Autodesk Inventor part; units mm, degrees
ref_plane "YZ Plane" through (0, 0, 0) normal (1, 0, 0) x (0, 1, 0)
ref_plane "XZ Plane" through (0, 0, 0) normal (0, 1, 0) x (-1, 0, 0)
ref_plane "XY Plane" through (0, 0, 0) normal (0, 0, 1) x (1, 0, 0)
sketch "Sketch1" plane through (0, 0, 0) normal (0, 1, 0) x (-1, 0, 0)
  line L0 (0, 0) -> (100, 0)
  line L1 (100, 0) -> (100, -180)
  line L2 (100, -180) -> (0, -180)
  line L3 (0, -180) -> (0, 0)
  dimension "d0" = 100
  dimension "d1" = 180
extrude "Extrusion1" add sketch "Sketch1" along normal blind 4
sketch "Sketch2" plane through (0, 4, 0) normal (0, 1, 0) x (1, 0, 0)
  line L0 (-100, 180) -> (-100, 0)
  line L1 (0, 180) -> (-100, 180)
  line L2 (-100, 0) -> (-96, 0)
  line L3 (-96, 0) -> (-96, 180)
  line L4 (-96, 180) -> (-100, 180)
  line L5 (-100, 180) -> (-100, 0)
  line L6 (0, 180) -> (-4, 180)
  line L7 (-4, 180) -> (-4, 0)
  line L8 (-4, 0) -> (0, 0)
  line L9 (0, 0) -> (0, 180)
  dimension "d4" = 4
  dimension "d5" = 4
extrude "Extrusion2" add sketch "Sketch2" along normal blind 5 contours L1 L9 L8 L7
sketch "Sketch3" plane through (0, 4, 0) normal (0, 1, 0) x (1, 0, 0)
  line L0 (-4, 180) -> (-4, 0)
  line L1 (-4, 0) -> (-34, 0)
  line L2 (-34, 0) -> (-34, 4)
  line L3 (-34, 4) -> (-4, 4)
  line L4 (-4, 4) -> (-4, 0)
  line L5 (-4, 180) -> (-100, 180)
  line L6 (-4, 180) -> (-34, 180)
  line L7 (-34, 180) -> (-34, 176)
  line L8 (-34, 176) -> (-4, 176)
  line L9 (-4, 176) -> (-4, 180)
  line L10 (-100, 0) -> (0, 0)
  line L11 (-100, 0) -> (-96, 0)
  line L12 (-96, 0) -> (-96, 180)
  line L13 (-96, 180) -> (-100, 180)
  line L14 (-100, 180) -> (-100, 0)
  point P0 (-4, 176)
  point P1 (-4, 4)
  dimension "d8" = 30
  dimension "d9" = 4
  dimension "d10" = 4
  dimension "d11" = 4
extrude "Extrusion3" add sketch "Sketch3" along normal blind 25 contours L0 L8 L7 L5 | L0 L1 L2 L3 | L12 L10 L14 L5
sketch "Sketch4" plane through (0, 29, 0) normal (0, 1, 0) x (1, 0, 0)
  line L0 (-100, 0) -> (-96, 0)
  line L1 (-96, 0) -> (-96, 180)
  line L2 (-96, 180) -> (-100, 180)
  line L3 (-100, 180) -> (-100, 0)
  line L4 (-4, 176) -> (-4, 180)
  line L5 (-4, 180) -> (-34, 180)
  line L6 (-34, 180) -> (-34, 176)
  line L7 (-34, 176) -> (-4, 176)
  line L8 (-34, 0) -> (-4, 0)
  line L9 (-34, 4) -> (-34, 0)
  line L10 (-34, 0) -> (-4, 0)
  line L11 (-4, 0) -> (-4, 4)
  line L12 (-4, 4) -> (-34, 4)
  line L13 (-100, 90) -> (-100, 145)
  line L14 (-100, 145) -> (-96, 145)
  line L15 (-96, 145) -> (-96, 35)
  line L16 (-96, 0) -> (-96, 180)
  line L17 (-96, 35) -> (-100, 35)
  line L18 (-100, 35) -> (-100, 90)
  line L19 (-4, 176) -> (-34, 176)
  line L20 (-19, 176) -> (-29, 176)
  line L21 (-29, 176) -> (-29, 180)
  line L22 (-29, 180) -> (-9, 180)
  line L23 (0, 180) -> (-100, 180)
  line L24 (-9, 180) -> (-9, 176)
  line L25 (-19, 176) -> (-9, 176)
  line L26 (-19, 4) -> (-29, 4)
  line L27 (-29, 4) -> (-29, 0)
  line L28 (-29, 0) -> (-9, 0)
  line L29 (-9, 0) -> (-9, 4)
  line L30 (-4, 4) -> (-34, 4)
  line L31 (-9, 4) -> (-19, 4)
  point P0 (0, 0)
  dimension "d14" = 55
  dimension "d15" = 110
  dimension "d16" = 10
  dimension "d17" = 20
extrude "Extrusion4" add sketch "Sketch4" along normal blind 3 contours L3 L14 L1 L17 | L5 L24 L7 L21 | L27 L12 L29 L8
sketch "Sketch5" plane through (0, 0, 0) normal (0, -1, 0) x (1, 0, 0)
  line L0 (-9, -4) -> (-29, -4)
  line L1 (-29, -4) -> (-29, 0)
  line L2 (-29, 0) -> (-9, 0)
  line L3 (-9, 0) -> (-9, -4)
  line L4 (-9, -180) -> (-29, -180)
  line L5 (-29, -180) -> (-29, -176)
  line L6 (-29, -176) -> (-9, -176)
  line L7 (-9, -176) -> (-9, -180)
  line L8 (-96, -35) -> (-96, -145)
  line L9 (-96, -145) -> (-100, -145)
  line L10 (-100, -145) -> (-100, -35)
  line L11 (-100, -35) -> (-96, -35)
  line L12 (-96, -180) -> (-96, 0)
  line L13 (-100, -35) -> (-96, -35)
  line L14 (-96, -35) -> (-96, -34.5)
  line L15 (-96, -34.5) -> (-100, -34.5)
  line L16 (-100, -34.5) -> (-100, -35)
  line L17 (-100, -145) -> (-96, -145)
  line L18 (-96, -145) -> (-96, -145.5)
  line L19 (-96, -145.5) -> (-100, -145.5)
  line L20 (-100, -145.5) -> (-100, -145)
  line L21 (-4, -176) -> (-34, -176)
  line L22 (-29, -180) -> (-29.5, -180)
  line L23 (-29.5, -180) -> (-29.5, -176)
  line L24 (-29.5, -176) -> (-29, -176)
  line L25 (-29, -176) -> (-29, -180)
  line L26 (-9, -176) -> (-8.5, -176)
  line L27 (-8.5, -176) -> (-8.5, -180)
  line L28 (-8.5, -180) -> (-9, -180)
  line L29 (-9, -180) -> (-9, -176)
  line L30 (-34, -4) -> (-4, -4)
  line L31 (-29, 0) -> (-29.5, 0)
  line L32 (-29.5, 0) -> (-29.5, -4)
  line L33 (-29.5, -4) -> (-29, -4)
  line L34 (-29, -4) -> (-29, 0)
  line L35 (-9, 0) -> (-8.5, 0)
  line L36 (-8.5, 0) -> (-8.5, -4)
  line L37 (-8.5, -4) -> (-9, -4)
  line L38 (-9, -4) -> (-9, 0)
  point P0 (0, 0)
  dimension "d22" = 0.5
  dimension "d23" = 0.5
  dimension "d24" = 0.5
  dimension "d25" = 0.5
  dimension "d26" = 0.5
  dimension "d27" = 0.5
extrude "Extrusion5" cut sketch "Sketch5" against normal blind 3.2
sketch "Sketch6" plane through (0, 32, 0) normal (0, 1, 0) x (1, 0, 0)
  line L0 (-126.3586, 197.6117) -> (20.3273, 197.6117)
  line L1 (20.3273, 197.6117) -> (20.3273, -20.388)
  line L2 (20.3273, -20.388) -> (-126.3586, -20.388)
  line L3 (-126.3586, -20.388) -> (-126.3586, 197.6117)
  point P0 (0, 0)
extrude "Extrusion6" cut sketch "Sketch6" against normal up to surface (28 mm away)
sketch "Sketch7" plane through (0, 4, 0) normal (0, 1, 0) x (1, 0, 0)
  line L0 (0, 180) -> (-100, 180)
  line L1 (-100, 0) -> (-100, 180)
  line L2 (-100, 0) -> (0, 0)
  line L3 (0, 180) -> (0, 0)
extrude "Extrusion7" add sketch "Sketch7" along normal blind 2
properties part number "caja_attiny"
CAD build for the part. Positions are in the model's coordinates, mm. A direction names the side the tool comes from. Give positions to 0.01 mm unless a question says otherwise; leave off trailing zeros. Order: outer loops, then holes, each group sorted by start corner. A loop starts at its lowest first (then second) coordinate and runs counter-clockwise, first axis right, second up. Notation, with made-up numbers: (67.5, 76.5) - (79.5, 76.5) arc R10 ccw to (79.5, 81.5) - close; hole circle Ø11 at (81, 68). An arc over 180 degrees is marked (long way). Write each question's results on one line, items separated by ' | '.
1. Probe L1, parallel to Z at x = -9, y = 1; L2, parallel to X at y = 0.45, z = -72. List the from-to ranges inside material, lowest first. Write a range as from..to.
Calculated:
L1: z = -176..-4 | L2: x = -96..0
2. Saw through at A-A on x = -15. List the corners of the cut face in (y, z), and give its area (3 significant figures).
Calculated:
outline: (0, -176) - (3.2, -176) - (3.2, -180) - (6, -180) - (6, 0) - (3.2, 0) - (3.2, -4) - (0, -4) - close | area: 1,050 mm2
3. Pull direction X, two halves, no side cores. Call faces 1 (the face through (-51, 6, -91)), 2 (the face through (-96, 2, -89)), 3 (the face through (-19, 3.2, -2)), 4 (the face through (0, 3, -91)): released by +X, released by -X, zero draft, split by the parting line, or undercut.
Calculated:
face 1: zero draft | face 2: released by -X | face 3: undercut | face 4: released by +X
4. Pin check, flat tips, straight feed: pin 1 (1 mm diameter, centred on x = -17, y = 1, fed in from +Z); pin 2 (2 mm diameter, centred on x = -98, z = -69, fed in from -Y); pin 3 (1 mm diameter, centred on x = -23, y = 2, fed in from -Z). Stop position of each tip, or through.
Calculated:
pin 1: stops at z = -4 | pin 2: stops at y = 3.2 | pin 3: stops at z = -176
5. Saw through at C-C on y = 2.05. List the corners of the cut face in (x, z).
Calculated:
outline: (-100, -180) - (-29.5, -180) - (-29.5, -176) - (-8.5, -176) - (-8.5, -180) - (0, -180) - (0, 0) - (-8.5, 0) - (-8.5, -4) - (-29.5, -4) - (-29.5, 0) - (-100, 0) - (-100, -34.5) - (-96, -34.5) - (-96, -145.5) - (-100, -145.5) - close
6. 3-axis set-ups, long thin cutter, end or side, ignore diameter. For faces 5 (the face through (-8.5, 2, -2)), 6 (the face through (-98, 3.2, -89)), 7 (the face through (-8.5, 2, -178)): which of +Z, -Z, +X, -X, +Y, -Y reach the whole face in a straight line?
Calculated:
face 5: +Z, -Y | face 6: -X, -Y | face 7: -Z, -Y
7. Saw through at B-B on z = -39. List the corners of the cut face in (x, y).
Calculated:
outline: (-100, 3.2) - (-96, 3.2) - (-96, 0) - (0, 0) - (0, 6) - (-100, 6) - close
